Verification items for the finished model (mm, model axes). A direction names the side the tool comes from. Round coordinates to 2 decimals unless told otherwise and drop trailing zeros. Write each loop counter-clockwise with the first axis right and the second up, starting at its lowest first coordinate (ties: lowest second). Pieces come first, ordered by that corner, then holes. Notation, with made-up numbers: M -34,47 L -2,47 A32 ccw -2,84 Z; hole C 46.25,82.25 d3. An arc over 180 degrees is marked long. Write each question's results on one line, items separated by ' | '.
from build123d import *

# Parameters (mm, degrees)
F1_DEPTH = 30
F2_R     = 5
F3_DEPTH = 3
F4_R     = 2.5
F5_DEPTH = 10
F6_R     = 2.5
F7_DEPTH = 25


with BuildPart() as f1:
    # F0 (on Front) → F1 (new body)
    with BuildSketch(Plane.XZ):
        Polygon((-35, 0), (0, 0), (35, 0), (35, 2), (15, 5), (0, 5), (-15, 5), (-35, 2), align=None)
    extrude(amount=F1_DEPTH)

    # F2 (on face) → F3 (cut)
    with BuildSketch(Plane.XY.offset(5)):
        with Locations((-7.5, -15)):
            Circle(F2_R)
        with Locations((7.5, -15)):
            Circle(F2_R)
    extrude(amount=-F3_DEPTH, mode=Mode.SUBTRACT)

    # F4 (on face) → F5 (cut)
    with BuildSketch(Plane.XY.offset(2)):
        with Locations((-7.5, -15)):
            Circle(F4_R)
    extrude(amount=-F5_DEPTH, mode=Mode.SUBTRACT)

    # F6 (on face) → F7 (cut)
    with BuildSketch(Plane.XY.offset(2)):
        with Locations((7.5, -15)):
            Circle(F6_R)
    extrude(amount=-F7_DEPTH, mode=Mode.SUBTRACT)


solid = f1.part
1) Sectioned sample at B-B, the plane x = -7.5. Record the cut outline in (y, z), and give its area (3 significant figures).
Calculated:
outline: M -30,0 L -17.5,0 L -17.5,2 L -20,2 L -20,5 L -30,5 Z; M -12.5,0 L 0,0 L 0,5 L -10,5 L -10,2 L -12.5,2 Z | area: 110 mm²
2) Sectioned sample at D-D, the plane y = -24.5. Record the cut outline in (x, z), and give its area (3 significant figures).
Calculated:
outline: M -35,0 L 35,0 L 35,2 L 15,5 L -15,5 L -35,2 Z | area: 290 mm²
3) Draft check along Y on faces 3 (the flat face through (0, 0, 2)), 4 (the cylindrical face through (9.81, -15.96, 1.01)), 5 (the flat face through (25.14, -14.79, 3.48)). Enter one of: pulls with the +Y half, pulls with the -Y half, needs draft (parallel to the pull), parting line crosses it, or undercut.
Calculated:
face 3: pulls with the +Y half | face 4: undercut | face 5: needs draft
4) Sectioned sample at C-C, the plane z = 1.3. Record the cut outline in (x, y), and give its area (3 significant figures).
Calculated:
outline: M -35,-30 L 35,-30 L 35,0 L -35,0 Z; hole C -7.5,-15 d5; hole C 7.5,-15 d5 | area: 2,060 mm²
5) Material ranges on line 1 (Y direction, x = 7.5, z = 0.55); line 2 (Z direction, x = -12, y = -15.75); line 3 (Y direction, x = -7.5, z = 4.2), recorded low to high. Write a range as [from, to].
Calculated:
line 1: y = [-30, -17.5], [-12.5, 0] | line 2: z = [0, 2] | line 3: y = [-30, -20], [-10, 0]
6) Depth check by flat-ended pin: P1, Ø8, axis at x = 7.5, y = -15, coming from the +Z side. Enter the tip coordinate at first touch or a pass-through.
Calculated:
P1: stops at z = 2
7) Sectioned sample at A-A, the plane y = -15. Record the cut outline in (x, z), and give its area (3 significant figures).
Calculated:
outline: M -35,0 L -10,0 L -10,2 L -12.5,2 L -12.5,5 L -15,5 L -35,2 Z; M -5,0 L 5,0 L 5,2 L 2.5,2 L 2.5,5 L -2.5,5 L -2.5,2 L -5,2 Z; M 10,0 L 35,0 L 35,2 L 15,5 L 12.5,5 L 12.5,2 L 10,2 Z | area: 210 mm²
8) Access from +Z, -Z, +X, -X, +Y, -Y to the whole of each face (thin tool, end or side, straight path). Record for faces 1 (the flat face through (-10, -16, 2)), 2 (the flat face through (0, -30, 2)).
Calculated:
face 1: +Z | face 2: +Z, -Z, +X, -X, -Y
